Build history of the part. All positions in model axes, mm. A direction names the side the tool comes from. Round coordinates to 2 decimals unless told otherwise and drop trailing zeros. Write each loop counter-clockwise with the first axis right and the second up, starting at its lowest first coordinate (ties: lowest second). Pieces come first, ordered by that corner, then holes. Notation, with made-up numbers: (38.5, 83) -> (62.5, 83) arc R18 ccw to (62.5, 93) -> close; hole circle Ø5 at (63.25, 21). An arc over 180 degrees is marked (long way). Answer in a Markdown table with one row per item.
```python
from build123d import *

# Parameters (mm, degrees)
F0_W     = 273.05
F0_H     = 114.3
F1_DEPTH = 19.05
F2_R     = 38.1
F3_DEPTH = 25.4
F5_DEPTH = 25.4


with BuildPart() as f1:
    # F0 (on Front) → F1 (new body)
    with BuildSketch(Plane.XZ):
        with Locations((136.525, 57.15)):
            Rectangle(F0_W, F0_H)
    extrude(amount=F1_DEPTH)

    # F2 (on face) → F3 (cut)
    with BuildSketch(Plane.XZ.offset(19.05)):
        with Locations((47.625, 50.8)):
            Circle(F2_R)
        with Locations((225.425, 50.8)):
            Circle(F2_R)
    extrude(amount=-F3_DEPTH, mode=Mode.SUBTRACT)

    # F4 (on face) → F5 (cut)
    with BuildSketch(Plane.XZ.offset(19.05)):
        with BuildLine():
            Line((177.8, 114.3), (95.25, 114.3))
            Line((95.25, 114.3), (95.25, 74.93))
            ThreePointArc((95.25, 74.93), (98.597769, 66.847769), (106.68, 63.5))
            Line((106.68, 63.5), (166.37, 63.5))
            ThreePointArc((166.37, 63.5), (174.452231, 66.847769), (177.8, 74.93))
            Line((177.8, 74.93), (177.8, 114.3))
        make_face()
    extrude(amount=-F5_DEPTH, mode=Mode.SUBTRACT)


solid = f1.part
```
Q1. Wall check: line 1 (X direction, y = -11, z = 50.5); line 2 (X direction, y = -16.25, z = 107.5); line 3 (X direction, y = -3.5, z = 69). Give the ranges that are in metal, low to high. Write a range as [from, to].
A:
| item | result |
|---|---|
| line 1 | [0, 9.53], [85.72, 187.33], [263.52, 273.05] |
| line 2 | [0, 95.25], [177.8, 273.05] |
| line 3 | [0, 14.15], [81.1, 96.91], [176.14, 191.95], [258.9, 273.05] |
Q2. Saw through at A-A on z = 101. Write the cut outline in (x, y), plus the area to 3 significant figures.
A:
| item | result |
|---|---|
| outline | (0, -19.05) -> (95.25, -19.05) -> (95.25, 0) -> (0, 0) -> close; (177.8, -19.05) -> (273.05, -19.05) -> (273.05, 0) -> (177.8, 0) -> close |
| area | 3,630 mm² |
Q3. Drop a flat-ended pin along its axis: P1, Ø5.5, axis at x = 136.5, y = -13, coming from the +Z side. Give the stop position or say it passes through.
A:
| item | result |
|---|---|
| P1 | z = 63.5 |
Q4. Two-plate mould, pull along X, no slides. Class faces 3 (the flat face through (135, -19.05, 58)), 4 (the cylindrical face through (195.19, -9.66, 27.62)), 5 (the flat face through (273.05, -9, 56)): released by +X, released by -X, zero draft, split by the parting line, or undercut.
A:
| item | result |
|---|---|
| face 3 | zero draft |
| face 4 | undercut |
| face 5 | released by +X |
Q5. Saw through at C-C on x = 66.5. Write the cut outline in (y, z), plus the area to 3 significant figures.
A:
| item | result |
|---|---|
| outline | (-19.05, 0) -> (0, 0) -> (0, 17.7) -> (-19.05, 17.7) -> close; (-19.05, 83.9) -> (0, 83.9) -> (0, 114.3) -> (-19.05, 114.3) -> close |
| area | 916 mm² |
Q6. Saw through at B-B on z = 50.8. Write the cut outline in (x, y) (3 decimals).
A:
| item | result |
|---|---|
| outline | (0, -19.05) -> (9.525, -19.05) -> (9.525, 0) -> (0, 0) -> close; (85.725, -19.05) -> (187.325, -19.05) -> (187.325, 0) -> (85.725, 0) -> close; (263.525, -19.05) -> (273.05, -19.05) -> (273.05, 0) -> (263.525, 0) -> close |
Q7. Which spindle directions (+Z, -Z, +X, -X, +Y, -Y) get a long thin tool onto all of the face, cutting with end or side? Do faces 1 (the flat face through (95.25, -10, 95)), 2 (the flat face through (47, -9, 114.3)). Say none if no direction does.
A:
| item | result |
|---|---|
| face 1 | +Z, +Y, -Y |
| face 2 | +Z, +X, -X, +Y, -Y |
Q8. Saw through at D-D on y = -13.5. Write the cut outline in (x, z) (3 decimals), plus the area to 3 significant figures.
A:
| item | result |
|---|---|
| outline | (0, 0) -> (273.05, 0) -> (273.05, 114.3) -> (177.8, 114.3) -> (177.8, 74.93) arc R11.43 cw to (166.37, 63.5) -> (106.68, 63.5) arc R11.43 cw to (95.25, 74.93) -> (95.25, 114.3) -> (0, 114.3) -> close; hole circle Ø76.2 at (47.625, 50.8); hole circle Ø76.2 at (225.425, 50.8) |
| area | 18,000 mm² |
